Geometry: final body of the model. Coordinates: model frame, mm. Face numbers are marked on the shaded views. A direction names the side the tool comes from. Round coordinates to 2 decimals unless told otherwise and drop trailing zeros. Order: outer loops, then holes, each group sorted by start corner. A loop starts at its lowest first (then second) coordinate and runs counter-clockwise, first axis right, second up. Notation, with made-up numbers: M -29.5,-37.5 L -8.5,-37.5 A25 cw -8.5,1.5 Z; hole C 48,-7 d1. An arc over 180 degrees is marked long. Return JSON: item names as keys, results as strings. Group by question number.
Q1. Cut plane A-A on y = 0. Output: boundary loops of the cut face in (x, z), and give its area (3 significant figures).
Q2. Ray query, probe 1 along Z at (x, y) = (43, -0.25); probe 2 along X at (y, z) = (0, 1.75). Return the intervals inside material, ascending.
Q3. Contact query for flat-ended pins moving along their axis: pin 1 (2 mm diameter, centred on x = 4.5, y = 4, fed in from -Z); pin 2 (4 mm diameter, centred on x = 2.5, z = -5, fed in from +Y); pin 3 (5 mm diameter, centred on x = 26.5, y = -2, fed in from +Z). Output: stop coordinate, or through.
Q4. Cut plane B-B on z = 0. Output: boundary loops of the cut face in (x, y).
Q5. Access query for the marked faces 1 and 2. Directions: +Z, -Z, +X, -X, +Y, -Y. A direction counts if a zero-diameter tool reaches every point of the face in a straight line with its end or side. Return the directions, or none.
Q6. Cut plane D-D on z = -5.5. Output: boundary loops of the cut face in (x, y), and give its area (3 significant figures).
Q7. Cut plane C-C on x = 60.5. Output: boundary loops of the cut face in (y, z) (1 decimal), and give its area (3 significant figures).
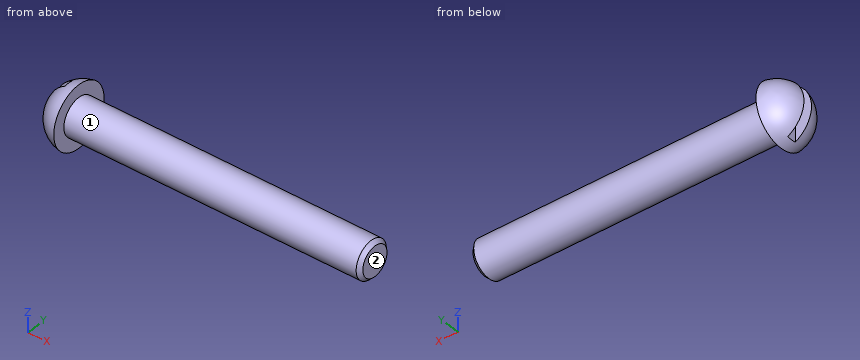
Autodesk Inventor part; units mm, degrees
ref_plane "IDS_WORKPLANE{1}" through (-6.9342, 0, 0) normal (1, 0, 0) x (0, 0, -1)
ref_plane "Work Plane2" through (41.275, 0, 0) normal (0, 0, -1) x (1, 0, 0)
ref_plane "YZ Plane" through (0, 0, 0) normal (1, 0, 0) x (0, 1, 0)
sketch "Sketch1" plane through (0, 0, 0) normal (0, 0, 1) x (1, 0, 0)
  line L0 (-6.9342, 0) -> (76.2, 0)
  line L1 (76.2, 0) -> (76.2, 4.7625)
  line L2 (76.2, 4.7625) -> (50.8, 4.7625)
  line L3 (50.8, 4.7625) -> (49.8475, 4.7625)
  line L4 (49.8475, 4.7625) -> (0, 4.7625)
  line L5 (0, 4.7625) -> (0, 7.9375)
  line L6 (-23.561, 0) -> (92.8268, 0)
  line L7 (0, -11.1125) -> (0, 11.1125)
  line L8 (0, -4.7625) -> (0, -7.9375) construction
  arc A0 (0, 7.9375) -> (0, -7.9375) centre (1.0759, 0) ccw
  line L9 (50.8, 4.7625) -> (0, 4.7625) construction
  dimension "d0" = 76.2
  dimension "d1" = 25.4
  dimension "d2" = 0.9525
  dimension "d3" = 6.9342
  dimension "d4" = 9.525
  dimension "d5" = 9.525
  dimension "d16" = 15.875
revolve "Body" add sketch "Sketch1" angle 360 about axis through (-6.9342, 0, 0) along (1, 0, 0) contours A0 L5 L7 L0 | L7 L4 L3 L2 L1 L0
ref_plane "IDS_WORKPLANE{1}" through (-6.9342, 0, 0) normal (1, 0, 0) x (0, 0, -1)
sketch "Sketch2" plane through (-6.9342, 0, 0) normal (1, 0, 0) x (0, 0, -1)
  line L0 (0, -11.1125) -> (0, 11.1125)
  line L1 (11.1125, 0) -> (-11.1125, 0)
  line L2 (-7.9375, 1.1938) -> (7.9375, 1.1938)
  line L3 (7.9375, 1.1938) -> (7.9375, -1.1938)
  line L4 (7.9375, -1.1938) -> (-7.9375, -1.1938)
  line L5 (-7.9375, -1.1938) -> (-7.9375, 1.1938)
  line L6 (-7.9375, 0) -> (7.9375, 0) construction
  line L7 (0, 1.1938) -> (0, -1.1938) construction
  circle A0 centre (0, 0) radius 7.9375
  dimension "d18" = 2.3876
extrude "Slot" cut sketch "Sketch2" along normal blind 4.2672 contours L4 A0 L1 L0 | L0 L1 A0 L4 | L4 L5 A0 | A0 L3 L4 | L1 A0 L2 L0 | L0 L2 A0 L1 | L5 L2 A0 | A0 L2 L3
thread "Thread"
chamfer "Chamfer1" distance 0.9462 distance2 0.9525 1 edges at (76.2, -4.7625, 0) measured on face at (76.2, 0.2765, -0.8749)
ref_plane "Work Plane2" through (41.275, 0, 0) normal (0, 0, -1) x (1, 0, 0)
equation "\"d0\" = NLG"
equation "\"d1\" = GEL"
equation "\"d2\" = GAL"
equation "\"d3\" = KOH"
equation "\"d4\" = GD"
equation "\"d5\" = BDM"
equation "\"d16\" = KOD"
equation "\"d18\" = SBR"
equation "\"d19\" = STI"
equation "\"d9\" = GEL"
equation "\"d11\" = -0.5 * SPD + 0.5 * GD"
equation "\"d12\" = GUL"
equation "\"GD\" = NND"
equation "\"NLG\" = 76.2"
equation "\"GEL\" = 25.4"
equation "\"KOD\" = 15.875"
equation "\"KOH\" = 6.9342"
equation "\"GAL\" = 0.9525"
equation "\"SPD\" = GD1"
equation "\"BDM\" = NND"
equation "\"GUL\" = GAL"
equation "\"STI\" = 4.2672"
equation "\"SBR\" = 2.3876"
equation "\"d17\" = -KOH"
equation "\"KR\" = KOH"
equation "\"THREADDIA\" = 9.525"
equation "\"TOA\" = 30deg"
equation "\"RR\" = 0.7874"
equation "\"NND\" = 9.525"
equation "\"GD1\" = 7.6327"
properties part number "ANSI B18.6.2 - 3/8-16 UNC - 3, SRHCSI" material "Steel, Mild"
Result sheet:
{
 "1": {"outline": "M -2.67,-7.08 A8.01 ccw 0,-7.94 L 0,-4.76 L 75.25,-4.76 L 76.2,-3.82 L 76.2,3.82 L 75.25,4.76 L 0,4.76 L 0,7.94 A8.01 ccw -2.67,7.08 Z", "area": "765 mm²"},
 "2": {"probe 1": "z = -4.76 to 4.76", "probe 2": "x = -2.67 to 76.2"},
 "3": {"pin 1": "stops at z = -3.7", "pin 2": "stops at y = 3.7", "pin 3": "stops at z = 4.76"},
 "4": {"outline": "M -6.84,-1.19 A8.01 ccw 0,-7.94 L 0,-4.76 L 75.25,-4.76 L 76.2,-3.82 L 76.2,3.82 L 75.25,4.76 L 0,4.76 L 0,7.94 A8.01 ccw -6.84,1.19 L -2.67,1.19 L -2.67,-1.19 Z"},
 "5": {"face 1": "+X", "face 2": "+Z, -Z, +X, +Y, -Y"},
 "6": {"outline": "M -4.62,-1.19 A5.82 ccw 0,-5.72 L 0,5.72 A5.82 ccw -4.62,1.19 L -2.67,1.19 L -2.67,-1.19 Z", "area": "35.9 mm²"},
 "7": {"outline": "C 0,0 d9.5", "area": "71.3 mm²"}
}
